Autodesk Inventor part; units mm, degrees
ref_plane "YZ Plane" through (0, 0, 0) normal (1, 0, 0) x (0, 1, 0)
ref_plane "XZ Plane" through (0, 0, 0) normal (0, 1, 0) x (-1, 0, 0)
ref_plane "XY Plane" through (0, 0, 0) normal (0, 0, 1) x (1, 0, 0)
sketch "Sketch1" plane through (0, 0, 0) normal (0, 0, 1) x (1, 0, 0)
  line L0 (0, 0) -> (38.1, 0)
  line L1 (38.1, 0) -> (38.1, 25.4)
  line L2 (38.1, 25.4) -> (0, 25.4)
  line L3 (0, 25.4) -> (0, 0)
  circle A0 centre (6.35, 12.7) radius 2.0828
  circle A1 centre (31.75, 12.7) radius 2.0828
  dimension "d0" = 38.1
  dimension "d1" = 25.4
  dimension "d2" = 4.1656
  dimension "d3" = 12.7
  dimension "d4" = 6.35
  dimension "d26" = 25.4
extrude "Plate1" add sketch "Sketch1" along normal blind 3.175
sketch "Sketch2" plane through (0, 25.4, 0) normal (0, 1, 0) x (1, 0, 0)
  line L0 (0, -3.175) -> (38.1, -3.175)
  line L1 (38.1, 0) -> (38.1, -3.175)
  line L2 (0, 0) -> (38.1, 0)
  line L3 (38.1, 0) -> (38.1, -184.15)
  line L4 (38.1, -184.15) -> (0, -184.15)
  line L5 (0, -184.15) -> (0, 0)
  circle A0 centre (6.35, -171.45) radius 2.4384
  line L6 (19.05, -184.15) -> (19.05, -3.175) construction
  circle A1 centre (31.75, -171.45) radius 2.4384
  circle A2 centre (7.6581, -49.0982) radius 2.4384
  circle A3 centre (7.6581, -36.3982) radius 2.4384
  circle A4 centre (30.4419, -49.0982) radius 2.4384
  circle A5 centre (30.4419, -36.3982) radius 2.4384
  line L7 (7.6581, -36.3982) -> (7.6581, -49.0982) construction
  dimension "d14" = 4.8768
  dimension "d15" = 184.15
  dimension "d16" = 12.7
  dimension "d17" = 12.7
  dimension "d21" = 12.7
  dimension "d22" = 11.3919
  dimension "d23" = 122.3518
extrude "Extrusion1" add sketch "Sketch2" along normal blind 3.175
equation "\"BendRadius\" = Thickness"
equation "\"BendReliefWidth\" = Thickness"
equation "\"BendReliefDepth\" = 0.5 * Thickness"
equation "\"CornerReliefSize\" = 4 * Thickness"
equation "\"MinimumRemnant\" = 2 * Thickness"
equation "\"TransitionRadius\" = BendRadius"
equation "\"JacobiRadiusSize\" = BendRadius"
equation "\"GapSize\" = Thickness"
equation "\"d13\" = BendRadius"
properties part number "Flange for 3-4 in Piston" material "Aluminum"
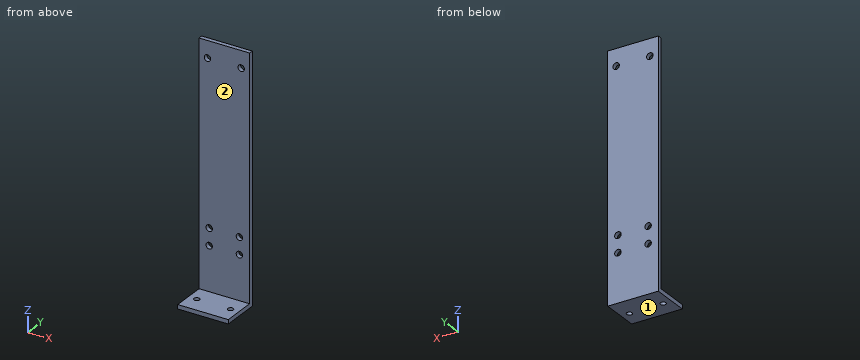
Work out the finished part from the listing and answer in its coordinate system (mm). Face numbers are marked on the shaded views. A direction names the side the tool comes from. Give positions to 0.01 mm unless a question says otherwise; leave off trailing zeros. Loops run counter-clockwise (first coordinate to the right, second up) from the corner with the lowest first, then second, coordinate; pieces in that order, holes last. Notation, with made-up numbers: (-29.75, 63.5) -> (-25.75, 63.5) arc R15 ccw to (-25.75, 85.5) -> close; hole circle Ø8 at (-28, -22). An arc over 180 degrees is marked (long way). Put each result on its own line as item: value. Start each with the question number.
Item 1: Which of the six approach directions +Z, -Z, +X, -X, +Y, -Y give full straight-line access (tool end or side, diameter ignored) to the marked faces 1 and 2?
Item 2: The part is cut by section C-C (z = 121.5). Give the vertices of the cut face in (x, y) (3 decimals), then the cut area to 3 significant figures.
Item 3: The part is cut by section B-B (y = 12.7). Give the vertices of the cut face in (x, z) (3 decimals).
Item 4: Each of these flat-tipped pins is pushed along its axis until it touches: P1, Ø7.5, axis at x = 22.5, y = 7, coming from the +Z side (3 decimals); P2, Ø10, axis at x = 31.5, z = 144, coming from the -Y side; P3, Ø5.5, axis at x = 31.75, z = 171.45, coming from the +Y side (3 decimals). Where does it stop, or does it pass through?
Item 5: The part is cut by section A-A (z = 171.45). Give the vertices of the cut face in (x, y) (3 decimals), then the cut area to 3 significant figures.
Item 6: Find the intervals of material crossed by L1, parallel to X at y = 27.9, z = 171.45; L2, parallel to Z at x = 6.35, y = 26.4; L3, parallel to Y at x = 27, z = 24 (3 decimals), in increasing order. Write a range as [from, to].
Answers below:
1. face 1: -Z, +X, -X, +Y, -Y
1. face 2: +Z, +X, -X, -Y
2. outline: (0, 25.4) -> (38.1, 25.4) -> (38.1, 28.575) -> (0, 28.575) -> close
2. area: 121 mm2
3. outline: (0, 0) -> (4.267, 0) -> (4.267, 3.175) -> (0, 3.175) -> close; (8.433, 0) -> (29.667, 0) -> (29.667, 3.175) -> (8.433, 3.175) -> close; (33.833, 0) -> (38.1, 0) -> (38.1, 3.175) -> (33.833, 3.175) -> close
4. P1: z = 3.175
4. P2: y = 25.4
4. P3: y = 28.575
5. outline: (0, 25.4) -> (3.912, 25.4) -> (3.912, 28.575) -> (0, 28.575) -> close; (8.788, 25.4) -> (29.312, 25.4) -> (29.312, 28.575) -> (8.788, 28.575) -> close; (34.188, 25.4) -> (38.1, 25.4) -> (38.1, 28.575) -> (34.188, 28.575) -> close
5. area: 90.0 mm2
6. L1: [0, 3.91], [8.79, 29.31], [34.19, 38.1]
6. L2: [0, 34.34], [38.46, 47.04], [51.16, 169.01], [173.89, 184.15]
6. L3: [25.4, 28.575]
